```python
from build123d import *

# Parameters (mm, degrees)
SKETCH1_R           = 31
BOSS_EXTRUDE1_DEPTH = 12
SKETCH2_R           = 3
CUT_EXTRUDE1_DEPTH  = 46.453272709
SKETCH3_R           = 3
BOSS_EXTRUDE2_DEPTH = 20


with BuildPart() as part:
    # Sketch1 → Boss-Extrude1 (new body)
    with BuildSketch(Plane(origin=(0, 0, 0), x_dir=(1, 0, 0), z_dir=(0, 1, 0))):
        with Locations(Location((0, 0, 0), (0, 0, 270))):
            Circle(SKETCH1_R)
    extrude(amount=BOSS_EXTRUDE1_DEPTH)

    # Sketch2 → Cut-Extrude1 (cut, through all)
    with BuildSketch(Plane(origin=(0, 12, 0), x_dir=(1, 0, 0), z_dir=(0, 1, 0))):
        with Locations(Location((0, 0, 0), (0, 0, 270))):
            Circle(SKETCH2_R)
    extrude(amount=-CUT_EXTRUDE1_DEPTH, mode=Mode.SUBTRACT)

    # Sketch3 → Boss-Extrude2 (add)
    with BuildSketch(Plane(origin=(0, 12, 0), x_dir=(1, 0, 0), z_dir=(0, 1, 0))):
        with Locations(Location((-14, 0, 0), (0, 0, 270))):
            Circle(SKETCH3_R)
    extrude(amount=BOSS_EXTRUDE2_DEPTH)


solid = part.part
```
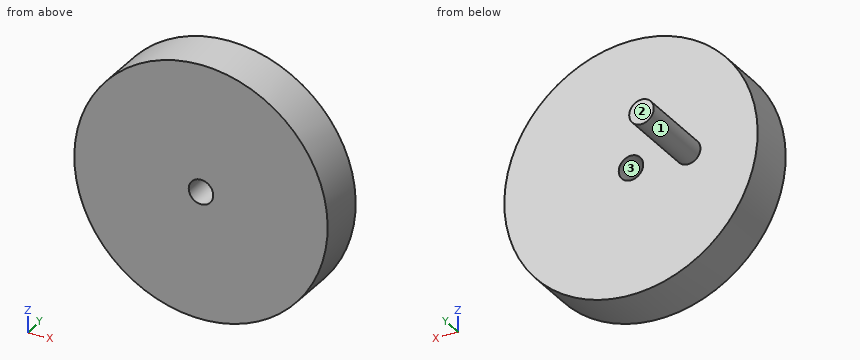
Here's how the part is built. I have some questions about the finished solid (model axes, mm). Face numbers are marked on the shaded views. Coordinates: 2 decimals unless noted, no trailing zeros. Loops run counter-clockwise (first coordinate to the right, second up) from the corner with the lowest first, then second, coordinate; pieces in that order, holes last. Notation, with made-up numbers: (81, -37) - (124, -37) arc R27 cw to (124, -5) - close; hole circle Ø5 at (57, 26). An arc over 180 degrees is marked (long way). Return JSON: item names as keys, results as strings. Group by question number.
Item 1: We'd pull the mould along Z, two halves only. Please class the marked faces 1, 2 and 3: +Z half, -Z half, draft (parallel to the pull), parting line (faces both ways), or undercut.
Item 2: If we section it at D-D on x = -14: Write out the boundary of the cut face in (y, z).
Item 3: If we section it at A-A on z = 0: Write out the boundary of the cut face in (x, y), and give its area (3 significant figures).
Item 4: If we section it at C-C on y = 10: Write out the boundary of the cut face in (x, z), and give its area (3 significant figures).
Item 5: Will these pins go through, and if not, where does the flat tip stop? P1, Ø10, axis at y = 11.5, z = 0, coming from the +X side; P2, Ø5.5, axis at x = 0, z = 0, coming from the -Y side; P3, Ø3, axis at x = 8, z = 13.5, coming from the +Y side; P4, Ø5, axis at y = 23.5, z = -2.5, coming from the -X side.
Item 6: If we section it at B-B on x = 0: Write out the boundary of the cut face in (y, z).
Item 7: I need wall thicknesses on line 1 (X direction, y = 5, z = 0); line 2 (Y direction, x = 5, z = -13.5); line 3 (X direction, y = 7, z = 16). Which ranges of each line are inside material? Lowest first, please. Write a range as from..to.
Calculated:
{
 "1": {"face 1": "parting line", "face 2": "draft", "face 3": "undercut"},
 "2": {"outline": "(0, -27.66) - (12, -27.66) - (12, -3) - (32, -3) - (32, 3) - (12, 3) - (12, 27.66) - (0, 27.66) - close"},
 "3": {"outline": "(-31, 0) - (-3, 0) - (-3, 12) - (-11, 12) - (-11, 32) - (-17, 32) - (-17, 12) - (-31, 12) - close; (3, 0) - (31, 0) - (31, 12) - (3, 12) - close", "area": "792 mm^2"},
 "4": {"outline": "circle Ø62 at (0, 0); hole circle Ø6 at (0, 0)", "area": "2,990 mm^2"},
 "5": {"P1": "stops at x = 31", "P2": "passes through", "P3": "stops at y = 12", "P4": "stops at x = -17"},
 "6": {"outline": "(0, -31) - (12, -31) - (12, -3) - (0, -3) - close; (0, 3) - (12, 3) - (12, 31) - (0, 31) - close"},
 "7": {"line 1": "x = -31..-3, 3..31", "line 2": "y = 0..12", "line 3": "x = -26.55..26.55"}
}
